Check sheet for the modelled part. Datum: model origin and axes. Units: mm. Face numbers are marked on the shaded views. A direction names the side the tool comes from. Round coordinates to 2 decimals unless told otherwise and drop trailing zeros. Write each loop counter-clockwise with the first axis right and the second up, starting at its lowest first coordinate (ties: lowest second). Pieces come first, ordered by that corner, then holes. Notation, with made-up numbers: M 87,36.25 L 142,36.25 A21 cw 142,66.25 Z; hole C -12,-32.75 d10. An arc over 180 degrees is marked long. One line per item, written item: value.
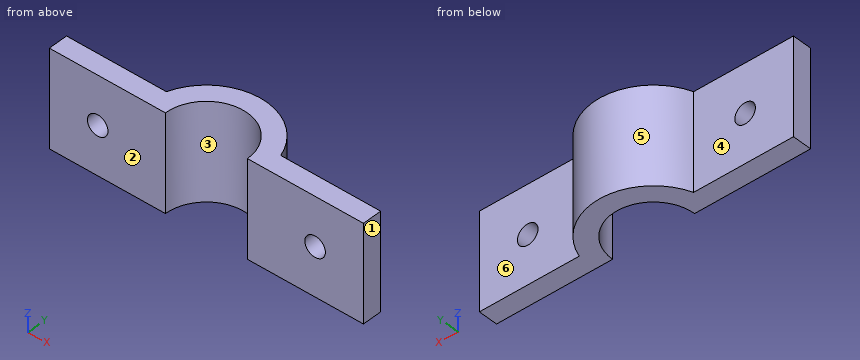
from build123d import *

# Parameters (mm, degrees)
BOSS_EXTRUDE1_DEPTH = 31.75
SKETCH3_R           = 3.3782
CUT_EXTRUDE1_DEPTH  = 7.35


with BuildPart() as part:
    # Sketch1 → Boss-Extrude1 (new body)
    with BuildSketch(Plane.XY):
        with BuildLine():
            Line((32.795198354, 6.35), (0, 6.35))
            Line((0, 6.35), (0, 0))
            Line((0, 0), (38.1, 0))
            ThreePointArc((38.1, 0), (51.562, 13.462), (65.024, 0))
            Line((65.024, 0), (103.124, 0))
            Line((103.124, 0), (103.124, 6.35))
            Line((103.124, 6.35), (70.328801646, 6.35))
            ThreePointArc((70.328801646, 6.35), (51.562, 19.812), (32.795198354, 6.35))
        make_face()
    extrude(amount=BOSS_EXTRUDE1_DEPTH)

    # Sketch3 → Cut-Extrude1 (cut, through all)
    with BuildSketch(Plane(origin=(0, 6.35, 0), x_dir=(1, 0, 0), z_dir=(0, 1, 0))):
        with Locations((15.875, -15.875)):
            Circle(SKETCH3_R)
        with Locations((87.249, -15.875)):
            Circle(SKETCH3_R)
    extrude(amount=-CUT_EXTRUDE1_DEPTH, mode=Mode.SUBTRACT)


solid = part.part
Q1. Sectioned sample at C-C on z = 29.5. Enter the section's corners in (x, y), and give its area (3 significant figures).
Completed:
outline: M 0,0 L 38.1,0 A13.46 cw 65.02,0 L 103.12,0 L 103.12,6.35 L 70.33,6.35 A19.81 ccw 32.8,6.35 L 0,6.35 Z
area: 739 mm^2
Q2. Draft check along X on the marked faces 1, 2 and 3. Enter one of: pulls with the +X half, pulls with the -X half, needs draft (parallel to the pull), parting line crosses it, or undercut.
Completed:
face 1: pulls with the +X half
face 2: needs draft
face 3: undercut
Q3. Depth check by flat-ended pin: P1, Ø1.5, axis at y = 11, z = 19.5, coming from the -X side; P2, Ø6, axis at x = 15.875, z = 15.875, coming from the -Y side; P3, Ø6, axis at y = 10.5, z = 6.5, coming from the +X side; P4, Ø11, axis at x = 87.249, z = 15.875, coming from the +Y side. Enter the tip coordinate at first touch or a pass-through.
Completed:
P1: x = 34.61
P2: through
P3: x = 69.9
P4: y = 6.35
Q4. Sectioned sample at B-B on x = 15. Enter the section's corners in (y, z).
Completed:
outline: M 0,0 L 6.35,0 L 6.35,12.61 L 0,12.61 Z; M 0,19.14 L 6.35,19.14 L 6.35,31.75 L 0,31.75 Z
Q5. Scan lines: line 1 (X direction, y = 5.25, z = 17.5); line 2 (Y direction, x = 86, z = 1.5); line 3 (X direction, y = 7, z = 24.5). Record each from-to range of solid material in increasing order. Write a range as [from, to].
Completed:
line 1: [0, 12.91], [18.84, 39.17], [63.96, 84.29], [90.21, 103.12]
line 2: [0, 6.35]
line 3: [33.03, 40.06], [63.06, 70.1]
Q6. Access from +Z, -Z, +X, -X, +Y, -Y to the whole of each face (thin tool, end or side, straight path). Record for the marked faces 4, 5 and 6.
Completed:
face 4: +Z, -Z, -X, +Y
face 5: +Z, -Z, +Y
face 6: +Z, -Z, +X, +Y
Q7. Sectioned sample at A-A on y = 5.25. Enter the section's corners in (x, z) (3 decimals).
Completed:
outline: M 0,0 L 39.166,0 L 39.166,31.75 L 0,31.75 Z; M 63.958,0 L 103.124,0 L 103.124,31.75 L 63.958,31.75 Z; hole C 15.875,15.875 d6.756; hole C 87.249,15.875 d6.756
Q8. Sectioned sample at D-D on y = 12.25. Enter the section's corners in (x, z), and give its area (3 significant figures).
Completed:
outline: M 35.99,0 L 45.98,0 L 45.98,31.75 L 35.99,31.75 Z; M 57.14,0 L 67.13,0 L 67.13,31.75 L 57.14,31.75 Z
area: 634 mm^2
